Here's how the part is built. I have some questions about the finished solid (model axes, mm). A direction names the side the tool comes from. Round coordinates to 2 decimals unless told otherwise and drop trailing zeros. Write each loop counter-clockwise with the first axis right and the second up, starting at its lowest first coordinate (ties: lowest second). Pieces come first, ordered by that corner, then holes. Notation, with made-up numbers: (47, 86) -> (66, 86) arc R23 ccw to (66, 123) -> close; hole circle Ø4 at (-37, 73.25). An arc over 180 degrees is marked (long way). Answer in a Markdown table with one row per item.
from build123d import *

# Parameters (mm, degrees)
SKETCH1_W             = 132
SKETCH1_H             = 65
MAIN_PLATE_BODY_DEPTH = 3
CHAMFER1_SIZE         = 8
MAIN_MOTOR_HOLE_R     = 19
MAIN_MOTOR_HOLE_R_2   = 2.6
MOTOR_HOLES_DEPTH     = 148.166572291
MOUNTING_SLOTS_DEPTH  = 148.166572291


with BuildPart() as part:
    # Sketch1 → Main Plate Body (new body)
    with BuildSketch(Plane(origin=(0, 0, 0), x_dir=(1, 0, 0), z_dir=(0, 1, 0))):
        with Locations((66, -32.5)):
            Rectangle(SKETCH1_W, SKETCH1_H)
    extrude(amount=MAIN_PLATE_BODY_DEPTH)

    # Chamfer1
    chamfer1_edges = [part.edges().sort_by_distance(p)[0] for p in [
        (0, 1.5, 0),
        (132, 1.5, 0),
        (132, 1.5, 65),
        (0, 1.5, 65),
    ]]
    chamfer(chamfer1_edges, length=CHAMFER1_SIZE)

    # Main Motor Hole → Motor Holes (cut, through all)
    with BuildSketch(Plane(origin=(0, 3, 0), x_dir=(1, 0, 0), z_dir=(0, 1, 0))):
        with Locations(Location((32.5, -32.5, 0), (0, 0, 270))):
            Circle(MAIN_MOTOR_HOLE_R)
        with Locations(Location((9, -56, 0), (0, 0, 270))):
            Circle(MAIN_MOTOR_HOLE_R_2)
        with Locations(Location((56, -56, 0), (0, 0, 90))):
            Circle(MAIN_MOTOR_HOLE_R_2)
        with Locations(Location((56, -9, 0), (0, 0, 270))):
            Circle(MAIN_MOTOR_HOLE_R_2)
        with Locations(Location((9, -9, 0), (0, 0, 90))):
            Circle(MAIN_MOTOR_HOLE_R_2)
    extrude(amount=-MOTOR_HOLES_DEPTH, mode=Mode.SUBTRACT)

    # T-Slot Mounting Slots → Mounting Slots (cut, through all)
    with BuildSketch(Plane(origin=(0, 3, 0), x_dir=(1, 0, 0), z_dir=(0, 1, 0))):
        with BuildLine():
            Line((122, -50.5), (79.8, -50.5))
            ThreePointArc((79.8, -50.5), (77.8, -52.5), (79.8, -54.5))
            Line((79.8, -54.5), (122, -54.5))
            ThreePointArc((122, -54.5), (124, -52.5), (122, -50.5))
        make_face()
        with BuildLine():
            Line((122, -10.5), (79.8, -10.5))
            ThreePointArc((79.8, -10.5), (77.8, -12.5), (79.8, -14.5))
            Line((79.8, -14.5), (122, -14.5))
            ThreePointArc((122, -14.5), (124, -12.5), (122, -10.5))
        make_face()
    extrude(amount=-MOUNTING_SLOTS_DEPTH, mode=Mode.SUBTRACT)


solid = part.part
1) I need wall thicknesses on line 1 (X direction, y = 1.05, z = 56); line 2 (Z direction, x = 119.5, y = 0.7); line 3 (X direction, y = 1.3, z = 32.5). Which ranges of each line are inside material? Lowest first, please. Write a range as [from, to].
Response:
| item | result |
|---|---|
| line 1 | x = [0, 6.4], [11.6, 53.4], [58.6, 132] |
| line 2 | z = [0, 10.5], [14.5, 50.5], [54.5, 65] |
| line 3 | x = [0, 13.5], [51.5, 132] |
2) I want a section at B-B, the plane z = 32.5. List the corners of the cut face in (x, y) for me.
Response:
| item | result |
|---|---|
| outline | (0, 0) -> (13.5, 0) -> (13.5, 3) -> (0, 3) -> close; (51.5, 0) -> (132, 0) -> (132, 3) -> (51.5, 3) -> close |
3) I want a section at A-A, the plane x = 32.5. List the corners of the cut face in (y, z) for me, and give its area (3 significant figures).
Response:
| item | result |
|---|---|
| outline | (0, 0) -> (3, 0) -> (3, 13.5) -> (0, 13.5) -> close; (0, 51.5) -> (3, 51.5) -> (3, 65) -> (0, 65) -> close |
| area | 81.0 mm^2 |
4) We'd pull the mould along Z, two halves only. Please class faces 1 (the face through (65, 1, 0)), 2 (the face through (124, 1.5, 12.5)), 3 (the face through (132, 1, 33)), 4 (the face through (65, 1, 65)): +Z half, -Z half, draft (parallel to the pull), parting line (faces both ways), or undercut.
Response:
| item | result |
|---|---|
| face 1 | -Z half |
| face 2 | undercut |
| face 3 | draft |
| face 4 | +Z half |
5) Which directions (+Z, -Z, +X, -X, +Y, -Y) give clear straight access to the entire face, cutting with the end or side of a thin tool? Please do faces 5 (the face through (77.8, 1.5, 12.5)), 6 (the face through (4, 1, 4)).
Response:
| item | result |
|---|---|
| face 5 | +Y, -Y |
| face 6 | -Z, -X, +Y, -Y |
6) For pin 1 (2 mm diameter, centred on x = 14.5, z = 36, fed in from +Y), with a flat end and sliding along its axis, tell me the tip position at first contact or that it passes through.
Response:
| item | result |
|---|---|
| pin 1 | stops at y = 3 |
7) I want a section at D-D, the plane x = 56. List the corners of the cut face in (y, z) for me, and give its area (3 significant figures).
Response:
| item | result |
|---|---|
| outline | (0, 0) -> (3, 0) -> (3, 6.4) -> (0, 6.4) -> close; (0, 11.6) -> (3, 11.6) -> (3, 53.4) -> (0, 53.4) -> close; (0, 58.6) -> (3, 58.6) -> (3, 65) -> (0, 65) -> close |
| area | 164 mm^2 |
8) I want a section at C-C, the plane y = 1.65. List the corners of the cut face in (x, z) for me.
Response:
| item | result |
|---|---|
| outline | (0, 8) -> (8, 0) -> (124, 0) -> (132, 8) -> (132, 57) -> (124, 65) -> (8, 65) -> (0, 57) -> close; hole circle Ø5.2 at (9, 9); hole circle Ø5.2 at (9, 56); hole circle Ø38 at (32.5, 32.5); hole circle Ø5.2 at (56, 9); hole circle Ø5.2 at (56, 56); hole (79.8, 10.5) -> (122, 10.5) arc R2 ccw to (122, 14.5) -> (79.8, 14.5) arc R2 ccw to start; hole (79.8, 50.5) -> (122, 50.5) arc R2 ccw to (122, 54.5) -> (79.8, 54.5) arc R2 ccw to start |
